Geometry: see drawing. Coordinates: mm, zero at the bounding-box minimum. A direction names the side the tool comes from. Coordinates: 2 decimals unless noted, no trailing zeros. Loops run counter-clockwise (first coordinate to the right, second up) from the corner with the lowest first, then second, coordinate; pieces in that order, holes last. Notation, with made-up numbers: (-2, 29.25) -> (53, 29.25) arc R30 cw to (53, 63.25) -> close; hole circle Ø1 at (-39.75, 25). An arc over 180 degrees is marked (long way). Put each result on its own line as item: value. Start each with the question number.
1) Cut plane C-C (z = 45.5). Return the cut outline in (x, y).
2) Cut plane D-D (y = 5.75). State how many separate pieces and enclosed holes the cut face has, plus the area to 3 significant figures.
3) Set-up query: the marked faces 3 and 4. Return all of +Z, -Z, +X, -X, +Y, -Y with unobstructed straight access to the full face (end or side cutting, diameter ignored); none if empty.
4) Cut plane A-A (z = 81). Return the cut outline in (x, y) (3 decimals).
5) Material intervals for L1, parallel to X at y = 9.75, z = 46.5 (1 decimal); L2, parallel to X at y = 3, z = 81 (3 decimals); L3, parallel to X at y = 9.25, z = 45.5, sorted ascending.
6) Pull-direction query (Z, two-part tool) for the marked faces 1 and 2; classes: pulls with the +Z half, pulls with the -Z half, needs draft (parallel to the pull), parting line crosses it, or undercut.
7) Cut plane B-B (x = 81). Return the cut outline in (y, z) (3 decimals).
8) Contact query for flat-ended pins moving along their axis: P1, Ø1, axis at x = 129.5, y = 6, coming from the -Z side; P2, Ø5, axis at x = 81, z = 10, coming from the +Y side; P3, Ø1, axis at x = 134, y = 5.5, coming from the +Z side; P4, Ø4, axis at y = 4, z = 100.5, coming from the -X side. Output: stop coordinate, or through.
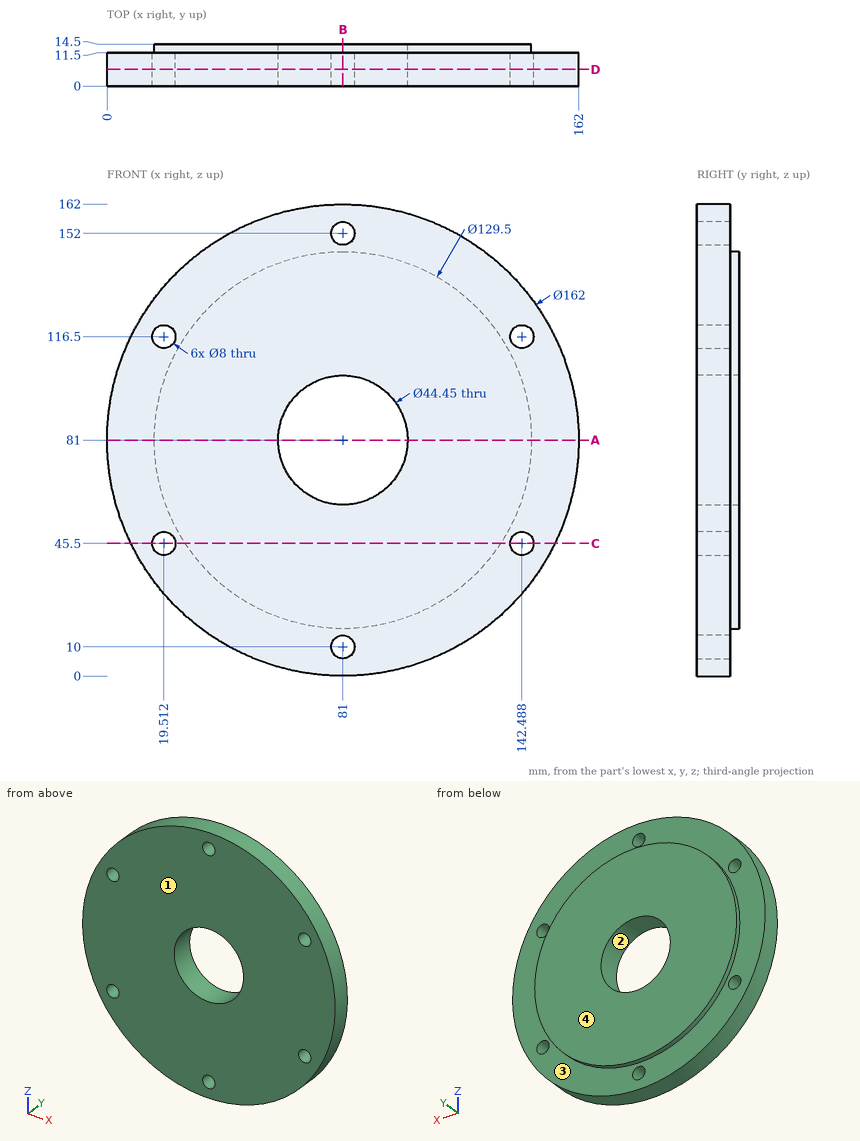
Results found:
1. outline: (8.19, 0) -> (15.51, 0) -> (15.51, 11.5) -> (8.19, 11.5) -> close; (23.51, 0) -> (138.49, 0) -> (138.49, 11.5) -> (135.15, 11.5) -> (135.15, 14.5) -> (26.85, 14.5) -> (26.85, 11.5) -> (23.51, 11.5) -> close; (146.49, 0) -> (153.81, 0) -> (153.81, 11.5) -> (146.49, 11.5) -> close
2. separate pieces: 1
2. enclosed holes: 7
2. area: 18,800 mm2
3. face 3: +Y
3. face 4: +Z, -Z, +X, -X, +Y
4. outline: (0, 0) -> (58.775, 0) -> (58.775, 14.5) -> (16.25, 14.5) -> (16.25, 11.5) -> (0, 11.5) -> close; (103.225, 0) -> (162, 0) -> (162, 11.5) -> (145.75, 11.5) -> (145.75, 14.5) -> (103.225, 14.5) -> close
5. L1: x = 7.7 to 15.6, 23.4 to 138.6, 146.4 to 154.3
5. L2: x = 0 to 58.775, 103.225 to 162
5. L3: x = 8.19 to 15.51, 23.51 to 138.49, 146.49 to 153.81
6. face 1: needs draft
6. face 2: undercut
7. outline: (0, 0) -> (11.5, 0) -> (11.5, 6) -> (0, 6) -> close; (0, 14) -> (11.5, 14) -> (11.5, 16.25) -> (14.5, 16.25) -> (14.5, 58.775) -> (0, 58.775) -> close; (0, 103.225) -> (14.5, 103.225) -> (14.5, 145.75) -> (11.5, 145.75) -> (11.5, 148) -> (0, 148) -> close; (0, 156) -> (11.5, 156) -> (11.5, 162) -> (0, 162) -> close
8. P1: stops at z = 15.75
8. P2: passes through
8. P3: stops at z = 142.68
8. P4: stops at x = 1.91
